```python
from build123d import *

# Parameters (mm, degrees)
F1_DEPTH = 1.3208
F2_R     = 3.175
F3_DEPTH = 25.4
F4_R     = 12.7


with BuildPart() as f1:
    # F0 (on Front) → F1 (new body)
    with BuildSketch(Plane.XZ):
        Polygon((0, 2514.6), (0, 0), (1244.6, 0), (1244.6, 2235.2), align=None)
    extrude(amount=F1_DEPTH)

    # F2 (on face) → F3 (cut)
    with BuildSketch(Plane.XZ.offset(1.3208)):
        with Locations((25.4, 2482.865801)):
            Circle(F2_R)
        with Locations((1219.2, 2214.869882)):
            Circle(F2_R)
        with Locations((399.952063, 2398.782685)):
            Circle(F2_R)
        with Locations((774.494473, 2314.701736)):
            Circle(F2_R)
        with Locations((1219.2, 25.4)):
            Circle(F2_R)
        with Locations((25.4, 25.4)):
            Circle(F2_R)
        with Locations((421.263099, 25.4)):
            Circle(F2_R)
        with Locations((794.35122, 25.4)):
            Circle(F2_R)
        with Locations((1219.2, 1120.134941)):
            Circle(F2_R)
        with Locations((1219.2, 1671.076059)):
            Circle(F2_R)
        with Locations((1219.2, 494.011074)):
            Circle(F2_R)
        with Locations((25.4, 1485.749841)):
            Circle(F2_R)
        with Locations((25.4, 1009.671807)):
            Circle(F2_R)
        with Locations((25.4, 566.66863)):
            Circle(F2_R)
        with Locations((25.4, 1981.021523)):
            Circle(F2_R)
    extrude(amount=-F3_DEPTH, mode=Mode.SUBTRACT)

    # F4
    f4_edges = [f1.edges().sort_by_distance(p)[0] for p in [
        (1244.6, -0.6604, 2235.2),
        (0, -0.6604, 2514.6),
        (1244.6, -0.6604, 0),
        (0, -0.6604, 0),
    ]]
    fillet(f4_edges, radius=F4_R)


solid = f1.part
```
Verification items for the finished model (mm, model axes). Coordinates: 2 decimals unless noted, no trailing zeros. Write each loop counter-clockwise with the first axis right and the second up, starting at its lowest first coordinate (ties: lowest second). Pieces come first, ordered by that corner, then holes. Notation, with made-up numbers: (-34, 7) - (16, 7) arc R10 ccw to (16, 25) - close; hole circle Ø11 at (4, 8.25). An arc over 180 degrees is marked (long way). Write item = value, one per line.
Q1. Cross-section at B-B (z = 2345). Enter the section's corners in (x, y), plus the area to 3 significant figures.
Answer:
outline = (0, -1.32) - (755.49, -1.32) - (755.49, 0) - (0, 0) - close
area = 998 mm²
Q2. Go/stop test with a flat-tipped pin: pin 1 Ø5.5 at (x, z) = (1219.2, 1120.13) entering from -Y. Record where the tip stops, or that it passes through.
Answer:
pin_1 = through
Q3. Material ranges on L1, parallel to X at y = -0.5, z = 2213; L2, parallel to Z at x = 1053.5, y = -0.4; L3, parallel to Z at x = 295, y = -0.1, recorded low to high. Write a range as from..to.
Answer:
L1 = 0..1216.63, 1221.77..1244.6
L2 = 0..2278.1
L3 = 0..2448.38
Q4. Mould release check, pull along Z, two halves, no side actions. Record for faces 1 (the face through (633.62, -0.65, 2372.36)), 2 (the face through (614, -1.321, 1273)): released by +Z, released by -Z, zero draft, split by the parting line, or undercut.
Answer:
face_1 = released by +Z
face_2 = zero draft
Q5. Cross-section at C-C (x = 194). Enter the section's corners in (y, z).
Answer:
outline = (-1.32, 0) - (0, 0) - (0, 2471.05) - (-1.32, 2471.05) - close
Q6. Cross-section at A-A (y = -0.65). Give the number of separate pieces and of enclosed holes in the cut face, plus the area to 3 significant figures.
Answer:
separate_pieces = 1
enclosed_holes = 15
area = 2,960,000 mm²
